Work out the finished part from the listing and answer in its coordinate system (mm). Face numbers are marked on the shaded views. A direction names the side the tool comes from. Give positions to 0.01 mm unless a question says otherwise; leave off trailing zeros. Order: outer loops, then holes, each group sorted by start corner. A loop starts at its lowest first (then second) coordinate and runs counter-clockwise, first axis right, second up. Notation, with made-up numbers: (-2, -15) -> (5, -15) arc R19 cw to (5, -4) -> close; hole circle Ø1 at (-31.75, 37.5). An arc over 180 degrees is marked (long way). Use a Markdown table: item, result. Add a question column.
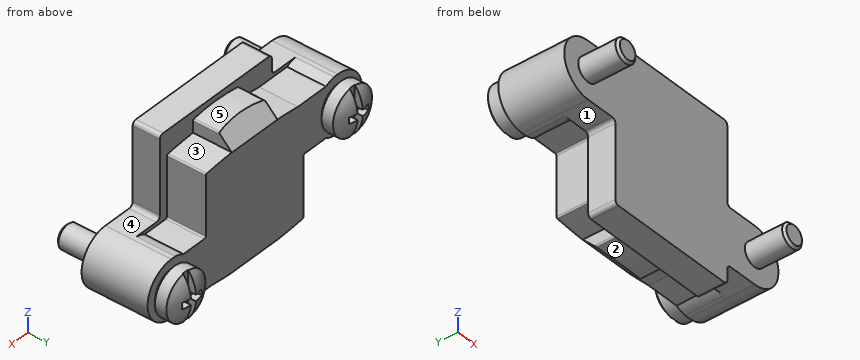
```python
from build123d import *

# Parameters (mm, degrees)
BOSS_EXTRUDE1_DEPTH     = 8.5
SKETCH2_W               = 40.53674955
SKETCH2_H               = 32.519038644
CUT_EXTRUDE1_DEPTH      = 5
CUT_EXTRUDE2_DEPTH      = 5
CUT_EXTRUDE2_DEPTH_BACK = 5
CUT_EXTRUDE3_DEPTH      = 5
CUT_EXTRUDE3_DEPTH_BACK = 5
CUT_EXTRUDE4_DEPTH      = 5
CUT_EXTRUDE5_DEPTH      = 5


with BuildPart() as part:
    # Sketch1 → Boss-Extrude1 (new body)
    with BuildSketch(Plane(origin=(0, 0, 0), x_dir=(1, 0, 0), z_dir=(0, 1, 0))):
        with BuildLine():
            Line((-12.8, -7.65), (-9.1, -7.65))
            ThreePointArc((-9.1, -7.65), (-8.746446609, -7.796446609), (-8.6, -8.15))
            Line((-8.6, -8.15), (-8.6, -9.6))
            ThreePointArc((-8.6, -9.6), (-8.453553391, -9.953553391), (-8.1, -10.1))
            Line((-8.1, -10.1), (8.1, -10.1))
            ThreePointArc((8.1, -10.1), (8.453553391, -9.953553391), (8.6, -9.6))
            Line((8.6, -9.6), (8.6, -0.18))
            ThreePointArc((8.6, -0.18), (8.755233406, 0.194766594), (9.13, 0.35))
            Line((9.13, 0.35), (12.8, 0.35))
            ThreePointArc((12.8, 0.35), (16.45, 4), (12.8, 7.65))
            Line((12.8, 7.65), (9.1, 7.65))
            ThreePointArc((9.1, 7.65), (8.746446609, 7.796446609), (8.6, 8.15))
            Line((8.6, 8.15), (8.6, 9.6))
            ThreePointArc((8.6, 9.6), (8.453553391, 9.953553391), (8.1, 10.1))
            Line((8.1, 10.1), (-8.1, 10.1))
            ThreePointArc((-8.1, 10.1), (-8.453553391, 9.953553391), (-8.6, 9.6))
            Line((-8.6, 9.6), (-8.6, 0.15))
            ThreePointArc((-8.6, 0.15), (-8.746446609, -0.203553391), (-9.1, -0.35))
            Line((-9.1, -0.35), (-12.8, -0.35))
            ThreePointArc((-12.8, -0.35), (-16.45, -4), (-12.8, -7.65))
        make_face()
    extrude(amount=BOSS_EXTRUDE1_DEPTH)

    # Sketch2 → Cut-Extrude1 (cut)
    with BuildSketch(Plane(origin=(0, 8.5, 0), x_dir=(1, 0, 0), z_dir=(0, 1, 0))):
        with Locations((0.049799447, -1.045788379)):
            Rectangle(SKETCH2_W, SKETCH2_H)
        with BuildLine():
            Line((-10.942582438, -7.2), (-6.658387125, -7.2))
            ThreePointArc((-6.658387125, -7.2), (-5.080966469, -7.35507325), (-3.5, -7.468425178))
            Line((-3.5, -7.468425178), (-3.5, -8.931694617))
            ThreePointArc((-3.5, -8.931694617), (-3.452752523, -9.060794062), (-3.333333333, -9.128897276))
            ThreePointArc((-3.333333333, -9.128897276), (0, -9.408631332), (3.333333333, -9.128897276))
            ThreePointArc((3.333333333, -9.128897276), (3.452752523, -9.060794062), (3.5, -8.931694617))
            Line((3.5, -8.931694617), (3.5, -7.468425178))
            ThreePointArc((3.5, -7.468425178), (5.414980187, -7.325745819), (7.324413769, -7.12185882))
            ThreePointArc((7.324413769, -7.12185882), (7.449804462, -7.055863448), (7.5, -6.923354493))
            Line((7.5, -6.923354493), (7.5, 0.6))
            ThreePointArc((7.5, 0.6), (7.558578644, 0.741421356), (7.7, 0.8))
            Line((7.7, 0.8), (10.942582438, 0.8))
            ThreePointArc((10.942582438, 0.8), (16.5, 4), (10.942582438, 7.2))
            Line((10.942582438, 7.2), (6.658387125, 7.2))
            ThreePointArc((6.658387125, 7.2), (5.080966469, 7.35507325), (3.5, 7.468425178))
            Line((3.5, 7.468425178), (3.5, 8.931694617))
            ThreePointArc((3.5, 8.931694617), (3.452752508, 9.060794079), (3.333333288, 9.128897284))
            ThreePointArc((3.333333288, 9.128897284), (-2.3e-08, 9.408631332), (-3.333333333, 9.128897276))
            ThreePointArc((-3.333333333, 9.128897276), (-3.452752523, 9.060794062), (-3.5, 8.931694617))
            Line((-3.5, 8.931694617), (-3.5, 7.468425178))
            ThreePointArc((-3.5, 7.468425178), (-5.414980187, 7.325745819), (-7.324413769, 7.12185882))
            ThreePointArc((-7.324413769, 7.12185882), (-7.449804462, 7.055863448), (-7.5, 6.923354493))
            Line((-7.5, 6.923354493), (-7.5, -0.6))
            ThreePointArc((-7.5, -0.6), (-7.558578644, -0.741421356), (-7.7, -0.8))
            Line((-7.7, -0.8), (-10.942582438, -0.8))
            ThreePointArc((-10.942582438, -0.8), (-16.5, -4), (-10.942582438, -7.2))
        make_face(mode=Mode.SUBTRACT)
    extrude(amount=-CUT_EXTRUDE1_DEPTH, mode=Mode.SUBTRACT)

    # Sketch3 → Cut-Extrude2 (cut, two sides)
    with BuildSketch(Plane(origin=(0, 0, 0), x_dir=(0, 0, -1), z_dir=(1, 0, 0))) as cut_extrude2_sk:
        Polygon((7.45, 8.5), (9.45, 6.5), (9.45, 8.5), align=None)
    extrude(amount=CUT_EXTRUDE2_DEPTH, mode=Mode.SUBTRACT)
    extrude(cut_extrude2_sk.sketch, amount=-CUT_EXTRUDE2_DEPTH_BACK, mode=Mode.SUBTRACT)

    # Sketch4 → Cut-Extrude3 (cut, two sides)
    with BuildSketch(Plane(origin=(0, 0, 0), x_dir=(0, 0, -1), z_dir=(1, 0, 0))) as cut_extrude3_sk:
        Polygon((-9.45, 6.5), (-7.45, 8.5), (-9.45, 8.5), align=None)
    extrude(amount=CUT_EXTRUDE3_DEPTH, mode=Mode.SUBTRACT)
    extrude(cut_extrude3_sk.sketch, amount=-CUT_EXTRUDE3_DEPTH_BACK, mode=Mode.SUBTRACT)

    # Sketch5 → Revolve1 (revolve)
    with BuildSketch(Plane.XY.offset(4)):
        with BuildLine():
            Line((-12.8, 8.5), (-15.3, 8.5))
            ThreePointArc((-15.3, 8.5), (-15.182842712, 8.782842712), (-14.9, 8.9))
            Line((-14.9, 8.9), (-12.8, 8.9))
            Line((-12.8, 8.9), (-12.8, 8.5))
        make_face()
    revolve(axis=Axis((-12.8, 8.9, 4), (0, -1, 0)))

    # Sketch6 → Revolve2 (revolve)
    with BuildSketch(Plane.XY.offset(-4)):
        with BuildLine():
            Line((12.8, 8.5), (10.3, 8.5))
            ThreePointArc((10.3, 8.5), (10.417157288, 8.782842712), (10.7, 8.9))
            Line((10.7, 8.9), (12.8, 8.9))
            Line((12.8, 8.9), (12.8, 8.5))
        make_face()
    revolve(axis=Axis((12.8, 8.9, -4), (0, -1, 0)))

    # Sketch7 → Cut-Revolve1 (revolve, cut)
    with BuildSketch(Plane.XY.offset(4)):
        with BuildLine():
            Line((-12.8, 0), (-14.3, 0))
            Line((-14.3, 0), (-14.3, 4.125))
            Line((-14.3, 4.125), (-14.175, 4.25))
            Line((-14.175, 4.25), (-14.3, 4.375))
            Line((-14.3, 4.375), (-14.3, 8.5))
            ThreePointArc((-14.3, 8.5), (-14.417157288, 8.782842712), (-14.7, 8.9))
            Line((-14.7, 8.9), (-12.8, 8.9))
            Line((-12.8, 8.9), (-12.8, 0))
        make_face()
    revolve(axis=Axis((-12.8, 8.9, 4), (0, -1, 0)), mode=Mode.SUBTRACT)

    # Sketch8 → Cut-Revolve2 (revolve, cut)
    with BuildSketch(Plane.XY.offset(-4)):
        with BuildLine():
            Line((12.8, 0), (11.3, 0))
            Line((11.3, 0), (11.3, 4.125))
            Line((11.3, 4.125), (11.425, 4.25))
            Line((11.425, 4.25), (11.3, 4.375))
            Line((11.3, 4.375), (11.3, 8.5))
            ThreePointArc((11.3, 8.5), (11.182842712, 8.782842712), (10.9, 8.9))
            Line((10.9, 8.9), (12.8, 8.9))
            Line((12.8, 8.9), (12.8, 0))
        make_face()
    revolve(axis=Axis((12.8, 8.9, -4), (0, -1, 0)), mode=Mode.SUBTRACT)

    # Sketch9 → Revolve3 (revolve)
    with BuildSketch(Plane.XY.offset(4)):
        with BuildLine():
            Line((-12.8, -5.1), (-13.9935, -5.1))
            Line((-13.9935, -5.1), (-14.3, -4.7935))
            Line((-14.3, -4.7935), (-14.3, 8.9))
            Line((-14.3, 8.9), (-15.8, 8.9))
            Line((-15.8, 8.9), (-15.8, 10.37))
            ThreePointArc((-15.8, 10.37), (-14.388759249, 11.136277748), (-12.8, 11.37))
            Line((-12.8, 11.37), (-12.8, -5.1))
        make_face()
    revolve(axis=Axis((-12.8, 11.37, 4), (0, -1, 0)))

    # Sketch10 → Revolve4 (revolve)
    with BuildSketch(Plane.XY.offset(-4)):
        with BuildLine():
            Line((12.8, -5.1), (11.6065, -5.1))
            Line((11.6065, -5.1), (11.3, -4.7935))
            Line((11.3, -4.7935), (11.3, 8.9))
            Line((11.3, 8.9), (9.8, 8.9))
            Line((9.8, 8.9), (9.8, 10.37))
            ThreePointArc((9.8, 10.37), (11.211240751, 11.136277748), (12.8, 11.37))
            Line((12.8, 11.37), (12.8, -5.1))
        make_face()
    revolve(axis=Axis((12.8, 11.37, -4), (0, -1, 0)))

    # Sketch11 → Cut-Extrude4 (cut)
    with BuildSketch(Plane(origin=(0, 10.3, 0), x_dir=(1, 0, 0), z_dir=(0, 1, 0))):
        Polygon((11.3, 3.6), (12.4, 3.6), (12.4, 1), (13.2, 1), (13.2, 3.6), (14.3, 3.6), (14.3, 4.4), (13.2, 4.4), (13.2, 7), (12.4, 7), (12.4, 4.4), (11.3, 4.4), align=None)
    extrude(amount=CUT_EXTRUDE4_DEPTH, mode=Mode.SUBTRACT)

    # Sketch12 → Cut-Extrude5 (cut)
    with BuildSketch(Plane(origin=(0, 10.3, 0), x_dir=(1, 0, 0), z_dir=(0, 1, 0))):
        Polygon((-14.3, -4.4), (-13.2, -4.4), (-13.2, -7), (-12.4, -7), (-12.4, -4.4), (-11.3, -4.4), (-11.3, -3.6), (-12.4, -3.6), (-12.4, -1), (-13.2, -1), (-13.2, -3.6), (-14.3, -3.6), align=None)
    extrude(amount=CUT_EXTRUDE5_DEPTH, mode=Mode.SUBTRACT)


solid = part.part
```
1) The part is cut by section C-C, the plane y = -1.5. Determine the outline of the cut face in (x, z), then the cut area to 3 significant figures.
2) The part is cut by section B-B, the plane z = 4. State how many separate pieces and enclosed holes the cut face has, then the cut area to 3 significant figures.
3) Straight lines are drawn through the part: line 1 (Y direction, x = -7.5, z = 6.25); line 2 (Z direction, x = 12, y = 1); line 3 (Z direction, x = -5.5, y = 4.75). For each, find the intervals that lie inside material, in ascending order.
4) Which of the six approach directions +Z, -Z, +X, -X, +Y, -Y give full straight-line access (tool end or side, diameter ignored) to the marked faces 1, 2, 3, 4 and 5?
5) Flat-ended cylindrical pins translate along their axes: pin 1 (1.8 mm diameter, centred on x = 11.5, y = 3.5, fed in from +Z); pin 2 (1 mm diameter, centred on x = 8.5, y = 5, fed in from +Z); pin 3 (0.5 mm diameter, centred on x = -13.5, y = 10.5, fed in from +Z); pin 4 (1.5 mm diameter, centred on y = -2.5, z = 7, fed in from +X). Find the tip coordinate at first contact, or state that the pin passes through.
6) The part is cut by section A-A, the plane y = 9.5. Determine the outline of the cut face in (x, z).
A:
| question | item | result |
|---|---|---|
| 1 | outline | circle Ø3 at (-12.8, 4); circle Ø3 at (12.8, -4) |
| 1 | area | 14.1 mm^2 |
| 2 | separate pieces | 1 |
| 2 | enclosed holes | 2 |
| 2 | area | 234 mm^2 |
| 3 | line 1 | 0 to 8.5 |
| 3 | line 2 | -7.65 to -0.35 |
| 3 | line 3 | -7.32 to 7.32 |
| 4 | face 1 | -Z, -X, +Y, -Y |
| 4 | face 2 | -Z, +Y |
| 4 | face 3 | +Z, +X, +Y |
| 4 | face 4 | +Z, +X, +Y, -Y |
| 4 | face 5 | +Z, +Y |
| 5 | pin 1 | z = -0.35 |
| 5 | pin 2 | z = -0.8 |
| 5 | pin 3 | z = 6.96 |
| 5 | pin 4 | through |
| 6 | outline | circle Ø6 at (-12.8, 4); circle Ø6 at (12.8, -4) |
